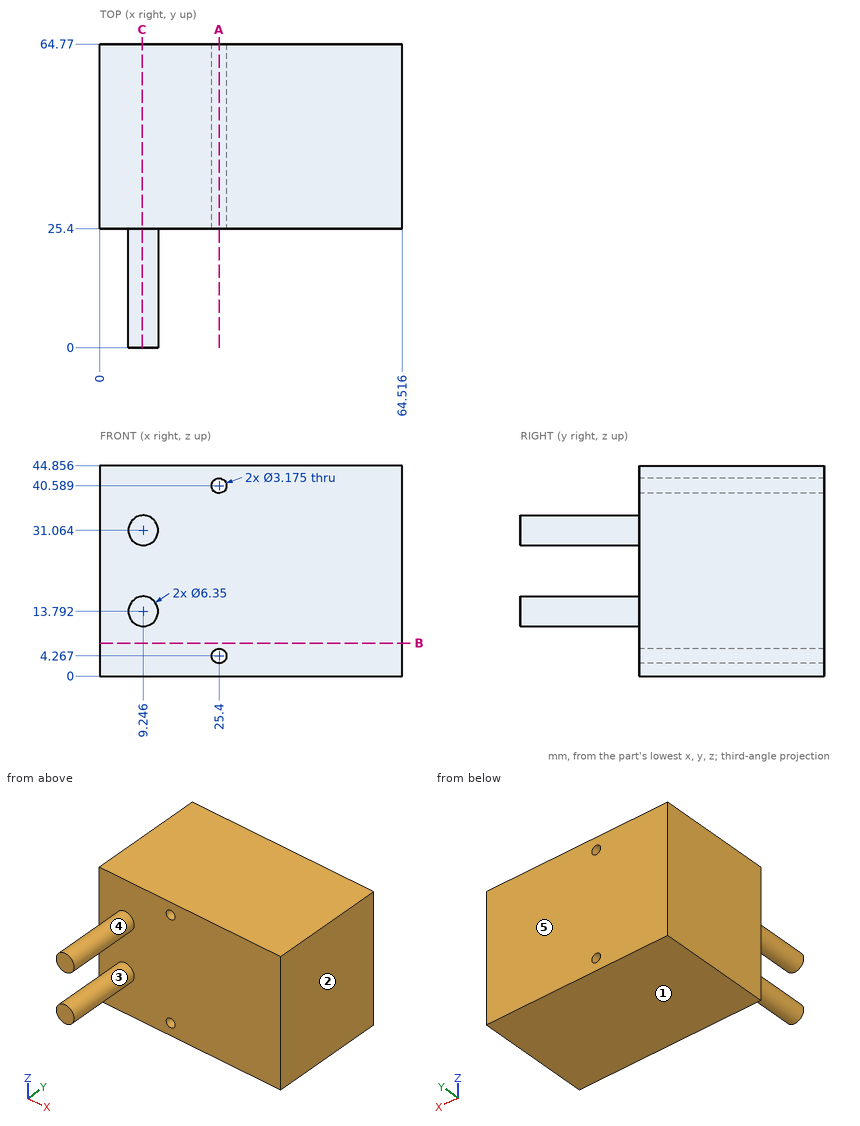
For this review, use the dimensioned drawing (mm, ordinates from the lowest corner) and the shaded views. A direction names the side the tool comes from. Give positions to 0.01 mm unless a question says otherwise; leave off trailing zeros. Write each loop counter-clockwise with the first axis right and the second up, starting at its lowest first coordinate (ties: lowest second). Pieces come first, ordered by that corner, then holes. Notation, with made-up numbers: M 80,79 L 113,79 A17 cw 113,103 Z; hole C 72.5,61.5 d7. An arc over 180 degrees is marked long. Write item = value, one per line. Start each with the question number.
Q1. For line 1 (Z direction, x = 25.4, y = 38) (1 decimal); line 2 (Z direction, x = 25, y = 44) (1 decimal); line 3 (Y direction, x = 34, z = 35.5), list the stretches that pass through material, from the lowest coordinate up.
Q2. Clearance check with flat-ended pins moving along their axes: pin 1 (2 mm diameter, centred on y = 15, z = 29, fed in from +X); pin 2 (5 mm diameter, centred on x = 49, z = 23, fed in from -Y); pin 3 (10 mm diameter, centred on x = 42.5, y = 17, fed in from -Z). State where each tip first meets the part, or that it passes through.
Q3. We need section B-B (z = 7). State the section outline as (x, y) points.
Q4. Mouldability with a two-part tool opening along Z and no side actions: class the marked faces 1, 2 and 3 as released by +Z, released by -Z, zero draft, split by the parting line, or undercut.
Q5. We need section C-C (x = 9). State the section outline as (y, z) points.
Q6. We need section A-A (x = 25.4). State the section outline as (y, z) points (1 decimal), plus the area to 3 significant figures.
Q7. Machinability: for the marked faces 4 and 5, which of the approach directions +Z, -Z, +X, -X, +Y, -Y give a long, thin tool a straight path to every point of the face, cutting with its end or side? Answer none if there is none.
Result set:
q1.line_1 = 0 to 2.7, 5.9 to 39, 42.2 to 44.9
q1.line_2 = 0 to 2.7, 5.8 to 39.1, 42.1 to 44.9
q1.line_3 = 25.4 to 64.77
q2.pin_1 = 12.24
q2.pin_2 = 25.4
q2.pin_3 = through
q3.outline = M 0,25.4 L 64.52,25.4 L 64.52,64.77 L 0,64.77 Z
q4.face_1 = released by -Z
q4.face_2 = zero draft
q4.face_3 = undercut
q5.outline = M 0,10.63 L 25.4,10.63 L 25.4,0 L 64.77,0 L 64.77,44.86 L 25.4,44.86 L 25.4,34.23 L 0,34.23 L 0,27.9 L 25.4,27.9 L 25.4,16.96 L 0,16.96 Z
q6.outline = M 25.4,0 L 64.8,0 L 64.8,2.7 L 25.4,2.7 Z; M 25.4,5.9 L 64.8,5.9 L 64.8,39 L 25.4,39 Z; M 25.4,42.2 L 64.8,42.2 L 64.8,44.9 L 25.4,44.9 Z
q6.area = 1,520 mm2
q7.face_4 = -Y
q7.face_5 = +Z, -Z, +X, -X, +Y
